```python
from build123d import *

# Parameters (mm, degrees)
F0_R     = 10.99621
F1_DEPTH = 25.4
F2_DEPTH = 41.91


with BuildPart() as f1:
    # F0 (on Front) → F1 (new body)
    with BuildSketch(Plane.XZ):
        with BuildLine():
            ThreePointArc((26.165782, 45.422908), (0, 71.588689), (-26.165782, 45.422908))
            Line((-26.165782, 45.422908), (-26.165782, -45.422908))
            ThreePointArc((-26.165782, -45.422908), (0, -19.257126), (26.165782, -45.422908))
            Line((26.165782, -45.422908), (26.165782, 45.422908))
        make_face()
        with Locations((0, 45.422908)):
            Circle(F0_R, mode=Mode.SUBTRACT)
        with BuildLine():
            ThreePointArc((26.165782, -45.422908), (0, -19.257126), (-26.165782, -45.422908))
            ThreePointArc((-26.165782, -45.422908), (0, -71.588689), (26.165782, -45.422908))
        make_face()
        with Locations((0, -45.422908)):
            Circle(F0_R, mode=Mode.SUBTRACT)
    extrude(amount=F1_DEPTH)

    # F0 (on Front) → F2 (join)
    with BuildSketch(Plane.XZ):
        with BuildLine():
            ThreePointArc((26.165782, -45.422908), (0, -19.257126), (-26.165782, -45.422908))
            ThreePointArc((-26.165782, -45.422908), (0, -71.588689), (26.165782, -45.422908))
        make_face()
        with Locations((0, -45.422908)):
            Circle(F0_R, mode=Mode.SUBTRACT)
    extrude(amount=-F2_DEPTH)

    # F3: F1 across face


with BuildPart() as f1_1:
    add(f1.part)
    add(f1.part.mirror(Plane(origin=(0, 41.91, -45.422908), x_dir=(1, 0, 0), z_dir=(0, 1, 0))))


solid = f1_1.part
```
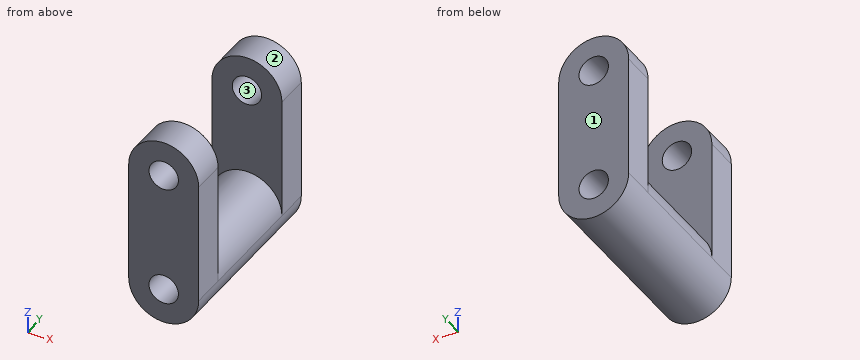
The listing builds one solid part. Answer for the finished solid, in the listing's coordinates (mm). Face numbers are marked on the shaded views. Coordinates: 2 decimals unless noted, no trailing zeros. Loops run counter-clockwise (first coordinate to the right, second up) from the corner with the lowest first, then second, coordinate; pieces in that order, holes last. Notation, with made-up numbers: M 80.25,59 L 121.25,59 A17 ccw 121.25,90 Z; hole C 40.5,9 d6. An arc over 180 degrees is marked long. Answer as a JSON object with one key per item and string values. Group by question number.
Item 1: Section B-B (y = 99.5) is taken. Write down the section's boundary in (x, z).
Item 2: Section D-D (z = -25) is taken. Write down the section's boundary in (x, y), and give its area (3 significant figures).
Item 3: Determine the mould class of the marked faces 1, 2 and 3 for opening direction X: +X half, -X half, draft (parallel to the pull), parting line (faces both ways), or undercut.
Item 4: Section A-A (x = 0) is taken. Write down the section's boundary in (y, z).
Item 5: Consider L1, parallel to Z at x = 0, y = -13.25; L2, parallel to Y at x = 2, z = 25; L3, parallel to X at y = 56, z = -46. Determine where each line is inside the solid, lowest interval first.
Item 6: Each of these flat-tipped pins is pushed along its axis until it touches: P1, Ø5, axis at x = -6, y = 16.5, coming from the +Z side; P2, Ø4, axis at y = 48, z = -52, coming from the +X side; P3, Ø4, axis at y = 23.5, z = -54, coming from the -X side; P4, Ø20, axis at x = 0, z = 45.42, coming from the -Y side. Where does it stop, or does it pass through?
Item 7: Section C-C (y = 34.5) is taken. Write down the section's boundary in (x, z).
Solved:
{
 "1": {"outline": "M -26.17,-45.42 A26.17 ccw 26.17,-45.42 L 26.17,45.42 A26.17 ccw -26.17,45.42 Z; hole C 0,-45.42 d21.99; hole C 0,45.42 d21.99"},
 "2": {"outline": "M -26.17,-25.4 L 26.17,-25.4 L 26.17,0 L 16.36,0 L 16.36,83.82 L 26.17,83.82 L 26.17,109.22 L -26.17,109.22 L -26.17,83.82 L -16.36,83.82 L -16.36,0 L -26.17,0 Z", "area": "5,400 mm2"},
 "3": {"face 1": "draft", "face 2": "parting line", "face 3": "undercut"},
 "4": {"outline": "M -25.4,-71.59 L 109.22,-71.59 L 109.22,-56.42 L -25.4,-56.42 Z; M -25.4,-34.43 L 109.22,-34.43 L 109.22,34.43 L 83.82,34.43 L 83.82,-19.26 L 0,-19.26 L 0,34.43 L -25.4,34.43 Z; M -25.4,56.42 L 0,56.42 L 0,71.59 L -25.4,71.59 Z; M 83.82,56.42 L 109.22,56.42 L 109.22,71.59 L 83.82,71.59 Z"},
 "5": {"L1": "z = -71.59 to -56.42, -34.43 to 34.43, 56.42 to 71.59", "L2": "y = -25.4 to 0, 83.82 to 109.22", "L3": "x = -26.16 to -10.98, 10.98 to 26.16"},
 "6": {"P1": "stops at z = -19.49", "P2": "stops at x = 25.76", "P3": "stops at x = -25.33", "P4": "passes through"},
 "7": {"outline": "M -26.17,-45.42 A26.17 ccw 26.17,-45.42 A26.17 ccw Z; hole C 0,-45.42 d21.99"}
}
